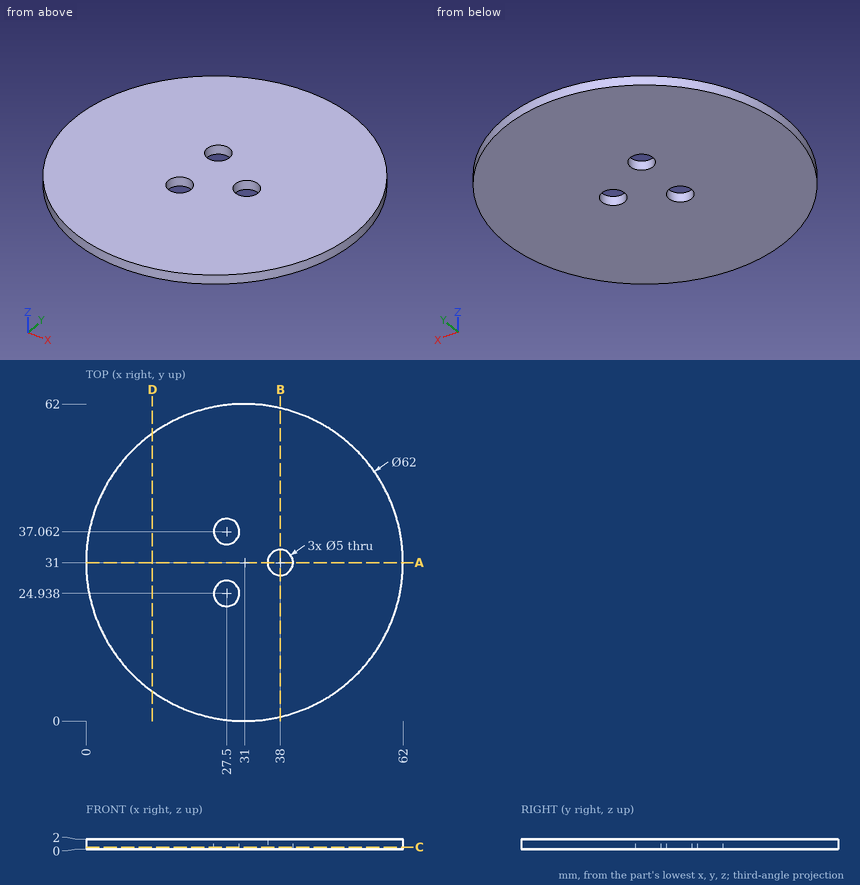
For this review, use the dimensioned drawing (mm, ordinates from the lowest corner) and the shaded views. Coordinates: 2 decimals unless noted, no trailing zeros. Order: outer loops, then holes, each group sorted by start corner. A loop starts at its lowest first (then second) coordinate and runs counter-clockwise, first axis right, second up. Notation, with made-up numbers: M -22,39.25 L 28,39.25 A26 cw 28,57.25 Z; hole C -4.5,-32.5 d9. An arc over 180 degrees is marked long. Answer as a JSON object with one key per item and string values. Group by question number.
1) Add section C-C, the plane z = 0.4. Write out the cut boundary in (x, y).
2) Add section A-A, the plane y = 31. Write out the cut boundary in (x, z), then the cut area to 3 significant figures.
3) Wall thickness on L1, parallel to Y at x = 27.5, z = 1.55; L2, parallel to X at y = 27, z = 0.95; L3, parallel to X at y = 26.5, z = 1.8: over which ranges is each line inside the solid? List them lowest first.
4) For pin 1 (4.5 mm diameter, centred on x = 27.5, y = 37.06, fed in from -Z), flat-tipped, find the tip position at first contact; note if it passes through.
5) Add section B-B, the plane x = 38. Write out the cut boundary in (y, z).
6) Add section D-D, the plane x = 13. Write out the cut boundary in (y, z), then the cut area to 3 significant figures.
Computed values:
{
 "1": {"outline": "C 31,31 d62; hole C 27.5,24.94 d5; hole C 27.5,37.06 d5; hole C 38,31 d5"},
 "2": {"outline": "M 0,0 L 35.5,0 L 35.5,2 L 0,2 Z; M 40.5,0 L 62,0 L 62,2 L 40.5,2 Z", "area": "114 mm^2"},
 "3": {"L1": "y = 0.2 to 22.44, 27.44 to 34.56, 39.56 to 61.8", "L2": "x = 0.26 to 26.09, 28.91 to 61.74", "L3": "x = 0.33 to 25.55, 29.45 to 61.67"},
 "4": {"pin 1": "passes through"},
 "5": {"outline": "M 0.8,0 L 28.5,0 L 28.5,2 L 0.8,2 Z; M 33.5,0 L 61.2,0 L 61.2,2 L 33.5,2 Z"},
 "6": {"outline": "M 5.76,0 L 56.24,0 L 56.24,2 L 5.76,2 Z", "area": "101 mm^2"}
}
